from build123d import *

# Parameters (mm, degrees)
F1_DEPTH = 37
F2_DEPTH = 37


with BuildPart() as f1:
    # F0 (on Right) → F1 (new body)
    with BuildSketch(Plane.YZ):
        Polygon((-600, -2050), (-589.859565, -1990), (-800, -1990), (-800, -2050), align=None)
        Polygon((0, -1990), (-589.859565, -1990), (-600, -2050), (0, -2050), align=None)
        Polygon((530.365877, -1990), (0, -1990), (0, -2050), (540.506312, -2050), align=None)
        Polygon((589.859565, -1990), (530.365877, -1990), (540.506312, -2050), (598.347846, -2040.224362), align=None)
        Polygon((800, -1990), (589.859565, -1990), (598.347846, -2040.224362), (600, -2050), (800, -2050), align=None)
        Polygon((598.347846, -2040.224362), (540.506312, -2050), (600, -2050), align=None)
    extrude(amount=F1_DEPTH)

    # F0 (on Right) → F2 (join)
    with BuildSketch(Plane.YZ):
        Polygon((188.075704, 35.298803), (236.291578, -249.989995), (295.785267, -249.989995), (245.917239, 45.074441), align=None)
        Polygon((295.785267, -249.989995), (236.291578, -249.989995), (530.365877, -1990), (589.859565, -1990), align=None)
        Polygon((589.859565, -1990), (530.365877, -1990), (540.506312, -2050), (598.347846, -2040.224362), align=None)
    extrude(amount=-F2_DEPTH)


solid = f1.part
Design review of the part built by this model. Coordinates are the model's own, in mm. A direction names the side the tool comes from. Round coordinates to 2 decimals unless told otherwise and drop trailing zeros. Loops run counter-clockwise (first coordinate to the right, second up) from the corner with the lowest first, then second, coordinate; pieces in that order, holes last. Notation, with made-up numbers: M 70,68.25 L 99,68.25 A10 ccw 99,86.25 Z; hole C -40,33 d2. An arc over 180 degrees is marked long. Answer as a JSON object with one key per item and string values.
Item 1: Clearance check with flat-ended pins moving along their axes: P1, Ø18, axis at y = 655, z = -2024, coming from the -X side; P2, Ø11, axis at x = 15.5, y = -129, coming from the +Z side; P3, Ø10, axis at x = -20, z = -291, coming from the +Y side. State where each tip first meets the part, or that it passes through.
Answer sheet:
{"P1": "stops at x = 0", "P2": "stops at z = -1990", "P3": "stops at y = 303.56"}
Item 2: We need section A-A on x = -19. Give the boundary of the cut face in (y, z).
Answer sheet:
{"outline": "M 188.08,35.3 L 540.51,-2050 L 598.35,-2040.22 L 245.92,45.07 Z"}
Item 3: Wall thickness on L1, parallel to Z at x = 3, y = 637.5; L2, parallel to Y at x = -27.5, z = -908; L3, parallel to Y at x = -7, z = -365.5: over which ranges is each line inside the solid? List them lowest first. Write a range as from..to.
Answer sheet:
{"L1": "z = -2050..-1990", "L2": "y = 347.5..406.99", "L3": "y = 255.81..315.31"}
Item 4: We need section C-C on z = -431. Give the boundary of the cut face in (x, y), and give its area (3 significant figures).
Answer sheet:
{"outline": "M -37,266.88 L 0,266.88 L 0,326.38 L -37,326.38 Z", "area": "2,200 mm^2"}
Item 5: We need section B-B on y = 78. Give the boundary of the cut face in (x, z).
Answer sheet:
{"outline": "M 0,-2050 L 37,-2050 L 37,-1990 L 0,-1990 Z"}
Item 6: Machinability: for faces 1 (the flat face through (0, -139, -2020)), 2 (the flat face through (0, 388, -968)), 3 (the flat face through (-37, 377, -998)), which of the approach directions +Z, -Z, +X, -X, +Y, -Y give a long, thin tool a straight path to every point of the face, cutting with its end or side? Answer none if there is none.
Answer sheet:
{"face 1": "-Z, -X, -Y", "face 2": "+Z, +X, +Y, -Y", "face 3": "+Z, -Z, -X, +Y, -Y"}
